Verification items for the finished model (mm, model axes). A direction names the side the tool comes from. Coordinates: 2 decimals unless noted, no trailing zeros. Order: outer loops, then holes, each group sorted by start corner. A loop starts at its lowest first (then second) coordinate and runs counter-clockwise, first axis right, second up. Notation, with made-up numbers: (65.25, -30.5) -> (109.25, -30.5) arc R21 cw to (109.25, 6.5) -> close; hole circle Ø5 at (78, 18). An arc over 180 degrees is marked (long way). Write item = value, one per line. Start each with the question number.
1. Thickness scan on line 1 along X through (y, z) = (29.5, 60); line 2 along Y through (x, z) = (66, 35); line 3 along Y through (x, z) = (14.5, 46.5). Record the ranges inside material, lowest first. Write a range as from..to.
2. Cross-section at C-C on y = 9. Record the cut outline in (x, z).
3. Cross-section at D-D on z = 33.5. Record the cut outline in (x, y).
4. Go/stop test with flat-tipped pins: P1, Ø5, axis at y = 49, z = 34.5, coming from the +X side; P2, Ø8.5, axis at x = 60, z = 7.5, coming from the +Y side; P3, Ø2, axis at x = 39.5, z = 43.5, coming from the +Y side; P4, Ø5, axis at x = 5.5, y = 64.5, coming from the +Z side. Record where each tip stops, or that it passes through.
5. Cross-section at B-B on x = 50.5. Record the cut outline in (y, z), plus the area to 3 significant figures.
6. Cross-section at A-A on z = 63. Record the cut outline in (x, y).
7. Release check for a two-part mould opening along X. For faces 1 (the flat face through (38.1, 57, 30)), 2 (the flat face through (35, 19, 38.1)), 3 (the flat face through (21.59, 57, 35)) record: +X half, -X half, draft (parallel to the pull), parting line (faces both ways), or undercut.
8. Set-up check for faces 4 (the flat face through (38.1, 8, 57)), 5 (the flat face through (35, 38.1, 19)), 6 (the flat face through (38.1, 57, 8)): record each of +Z, -Z, +X, -X, +Y, -Y from which the full face is reachable in a straight line by a thin tool's end or side.
Autodesk Inventor part; units mm, degrees
ref_plane "YZ Plane" through (0, 0, 0) normal (1, 0, 0) x (0, 1, 0)
ref_plane "XZ Plane" through (0, 0, 0) normal (0, 1, 0) x (-1, 0, 0)
ref_plane "XY Plane" through (0, 0, 0) normal (0, 0, 1) x (1, 0, 0)
sketch "Sketch1" plane through (0, 0, 0) normal (0, 0, 1) x (1, 0, 0)
  line L0 (0, 0) -> (38.1, 0)
  line L1 (38.1, 0) -> (38.1, 38.1)
  line L2 (38.1, 38.1) -> (0, 38.1)
  line L3 (0, 38.1) -> (0, 0)
  dimension "d0" = 38.1
  dimension "d1" = 38.1
extrude "Extrusion1" add sketch "Sketch1" along normal blind 38.1
sketch "Sketch2" plane through (0, 0, 38.1) normal (0, 0, 1) x (1, 0, 0)
  line L0 (6.35, 6.35) -> (32.004, 6.35)
  line L1 (32.004, 6.35) -> (32.004, 32.004)
  line L2 (32.004, 32.004) -> (6.35, 32.004)
  line L3 (6.35, 32.004) -> (6.35, 6.35)
  line L4 (38.1, 0) -> (38.1, 38.1)
  line L5 (0, 0) -> (38.1, 0)
  line L6 (38.1, 0) -> (38.1, 38.1)
  line L7 (38.1, 38.1) -> (0, 38.1)
  line L8 (0, 38.1) -> (0, 0)
  dimension "d4" = 25.654
  dimension "d5" = 25.654
extrude "Extrusion2" cut sketch "Sketch2" against normal blind 31.75 contours L3 L2 L1 L0
sketch "Sketch5" plane through (0, 0, 38.1) normal (0, 0, 1) x (1, 0, 0)
  line L0 (6.35, 6.35) -> (6.35, 32.004)
  line L1 (6.35, 6.35) -> (32.004, 6.35)
  line L2 (32.004, 6.35) -> (32.004, 32.004)
  line L3 (32.004, 32.004) -> (6.35, 32.004)
  line L4 (6.35, 32.004) -> (6.35, 6.35)
  line L5 (0, 0) -> (38.1, 0)
  line L6 (0, 0) -> (38.1, 0)
  line L7 (38.1, 0) -> (38.1, 38.1)
  line L8 (38.1, 38.1) -> (0, 38.1)
  line L9 (0, 38.1) -> (0, 0)
extrude "Extrusion4" add sketch "Sketch5" along normal blind 38.1
sketch "Sketch7" plane through (38.1, 0, 0) normal (1, 0, 0) x (0, 0, -1)
  line L0 (0, 0) -> (-76.2, 0)
  line L1 (0, 0) -> (-38.1, 0)
  line L2 (-38.1, 0) -> (-38.1, 38.1)
  line L3 (-38.1, 38.1) -> (0, 38.1)
  line L4 (0, 38.1) -> (0, 0)
  line L5 (-76.2, 6.35) -> (-6.35, 6.35)
  line L6 (-6.35, 6.35) -> (-32.004, 6.35)
  line L7 (-32.004, 6.35) -> (-32.004, 32.004)
  line L8 (-32.004, 32.004) -> (-6.35, 32.004)
  line L9 (-6.35, 32.004) -> (-6.35, 6.35)
  dimension "d16" = 38.1
  dimension "d17" = 38.1
  dimension "d20" = 25.654
  dimension "d21" = 25.654
extrude "Extrusion6" add sketch "Sketch7" along normal blind 38.1
sketch "Sketch9" plane through (38.1, 6.35, 6.35) normal (1, 0, 0) x (0, 0, -1)
  line L0 (-25.654, 0) -> (-25.654, 25.654)
  line L1 (0, 0) -> (0, 25.654)
  line L2 (-25.654, 0) -> (0, 0)
  line L3 (0, 0) -> (0, 25.654)
  line L4 (0, 25.654) -> (-25.654, 25.654)
  line L5 (-25.654, 25.654) -> (-25.654, 0)
  point P0 (6.35, -6.35)
extrude "Extrusion7" cut sketch "Sketch9" against normal blind 31.75
sketch "Sketch10" plane through (0, 38.1, 76.2) normal (0, 1, 0) x (1, 0, 0)
  line L0 (76.2, 69.85) -> (6.35, 69.85)
  line L1 (6.35, 69.85) -> (32.004, 69.85)
  line L2 (32.004, 69.85) -> (32.004, 44.196)
  line L3 (32.004, 44.196) -> (6.35, 44.196)
  line L4 (6.35, 44.196) -> (6.35, 69.85)
  line L5 (38.1, 38.1) -> (38.1, 0)
  line L6 (0, 76.2) -> (0, 0)
  line L7 (38.1, 38.1) -> (0, 38.1)
  line L8 (0, 38.1) -> (0, 76.2)
  line L9 (0, 76.2) -> (38.1, 76.2)
  line L10 (38.1, 76.2) -> (38.1, 38.1)
  point P0 (0, 38.1)
  dimension "d26" = 25.654
  dimension "d27" = 25.654
extrude "Extrusion8" add sketch "Sketch10" along normal blind 38.1
sketch "Sketch11" plane through (6.35, 38.1, 6.35) normal (0, 1, 0) x (1, 0, 0)
  line L0 (0, -25.654) -> (25.654, -25.654)
  line L1 (25.654, -25.654) -> (0, -25.654)
  line L2 (0, -25.654) -> (0, 0)
  line L3 (0, 0) -> (25.654, 0)
  line L4 (25.654, 0) -> (25.654, -25.654)
  point P0 (-6.35, 6.35)
extrude "Extrusion9" cut sketch "Sketch11" against normal blind 6.35
sketch "Sketch12" plane through (0, 76.2, 76.2) normal (0, 1, 0) x (1, 0, 0)
  line L0 (38.1, 55.88) -> (32.004, 55.88)
  line L1 (32.004, 55.88) -> (32.004, 58.42)
  line L2 (32.004, 58.42) -> (38.1, 58.42)
  line L3 (38.1, 58.42) -> (38.1, 55.88)
  point P0 (0, 76.2)
  dimension "d32" = 6.096
  dimension "d33" = 2.54
extrude "Extrusion10" cut sketch "Sketch12" against normal blind 38.1
sketch "Sketch13" plane through (76.2, 38.1, 38.1) normal (0, 1, 0) x (1, 0, 0)
  line L0 (0, 31.75) -> (0, 6.096)
  line L1 (-44.196, 17.78) -> (0, 17.78)
  line L2 (0, 17.78) -> (0, 20.32)
  line L3 (0, 20.32) -> (-44.196, 20.32)
  line L4 (-44.196, 20.32) -> (-44.196, 17.78)
  point P0 (-76.2, 38.1)
  dimension "d36" = 2.54
extrude "Extrusion11" cut sketch "Sketch13" against normal blind 6.35
sketch "Sketch15" plane through (0, 76.2, 76.2) normal (0, 1, 0) x (1, 0, 0)
  line L0 (17.78, 38.1) -> (20.32, 38.1)
  line L1 (20.32, 38.1) -> (20.32, 44.196)
  line L2 (20.32, 44.196) -> (17.78, 44.196)
  line L3 (17.78, 44.196) -> (17.78, 38.1)
  point P0 (0, 76.2)
  dimension "d39" = 2.54
  dimension "d40" = 6.096
extrude "Extrusion12" cut sketch "Sketch15" against normal blind 38.1
sketch "Sketch16" plane through (0, 38.1, 76.2) normal (0, 1, 0) x (1, 0, 0)
  line L0 (20.32, 44.196) -> (20.32, 38.1)
  line L1 (0, 0) -> (38.1, 0)
  line L2 (20.32, 44.196) -> (17.78, 44.196)
  line L3 (17.78, 44.196) -> (17.78, 0)
  line L4 (17.78, 0) -> (20.32, 0)
  line L5 (20.32, 0) -> (20.32, 44.196)
  point P0 (0, 76.2)
  dimension "d43" = 2.54
extrude "Extrusion13" cut sketch "Sketch16" against normal blind 6.35
sketch "Sketch17" plane through (38.1, 0, 76.2) normal (1, 0, 0) x (0, 0, -1)
  line L0 (38.1, 0) -> (38.1, 38.1)
  line L1 (0, 17.78) -> (38.1, 17.78)
  line L2 (38.1, 17.78) -> (38.1, 20.32)
  line L3 (38.1, 20.32) -> (0, 20.32)
  line L4 (0, 20.32) -> (0, 17.78)
  point P0 (76.2, 0)
  dimension "d46" = 2.54
extrude "Extrusion14" cut sketch "Sketch17" against normal blind 6.35
sketch "Sketch18" plane through (38.1, 0, 38.1) normal (0, 0, 1) x (1, 0, 0)
  line L0 (0, 17.78) -> (38.1, 17.78)
  line L1 (38.1, 17.78) -> (38.1, 20.32)
  line L2 (38.1, 20.32) -> (0, 20.32)
  line L3 (0, 20.32) -> (0, 17.78)
  point P0 (-38.1, 0)
  dimension "d49" = 38.1
  dimension "d50" = 2.54
extrude "Extrusion15" cut sketch "Sketch18" against normal blind 6.35
sketch "Sketch20" plane through (38.1, 38.1, 38.1) normal (0, 0, 1) x (1, 0, 0)
  line L0 (-17.78, -6.096) -> (-17.78, 38.1)
  line L1 (0, 0) -> (-17.78, 0)
  line L2 (-17.78, 38.1) -> (-16.51, 38.1)
  line L3 (-16.51, 38.1) -> (-16.51, 0)
  line L4 (-16.51, 0) -> (-17.78, 0)
  line L5 (-17.78, 0) -> (-17.78, 38.1)
  point P0 (-38.1, -38.1)
  dimension "d53" = 1.27
extrude "Extrusion16" cut sketch "Sketch20" against normal blind 6.35
sketch "Sketch21" plane through (38.1, 38.1, 76.2) normal (0, 1, 0) x (1, 0, 0)
  line L0 (-17.78, 0) -> (-17.78, 44.196)
  line L1 (0, 0) -> (-17.78, 0)
  line L2 (-17.78, 44.196) -> (-16.51, 44.196)
  line L3 (-16.51, 44.196) -> (-16.51, 0)
  line L4 (-16.51, 0) -> (-17.78, 0)
  line L5 (-17.78, 0) -> (-17.78, 44.196)
  point P0 (-38.1, 76.2)
  dimension "d56" = 1.27
extrude "Extrusion17" cut sketch "Sketch21" against normal blind 6.35
sketch "Sketch23" plane through (0, 38.1, 38.1) normal (0, 0, 1) x (1, 0, 0)
  line L0 (17.78, 0) -> (17.78, 38.1)
  line L1 (17.78, 0) -> (0, 0)
  line L2 (17.78, 38.1) -> (16.51, 38.1)
  line L3 (16.51, 38.1) -> (16.51, 0)
  line L4 (16.51, 0) -> (17.78, 0)
  line L5 (17.78, 0) -> (17.78, 38.1)
  point P0 (0, -38.1)
  dimension "d59" = 1.27
extrude "Extrusion18" cut sketch "Sketch23" against normal blind 6.35
sketch "Sketch24" plane through (0, 38.1, 76.2) normal (0, 1, 0) x (1, 0, 0)
  line L0 (17.78, 44.196) -> (17.78, 0)
  line L1 (17.78, 0) -> (0, 0)
  line L2 (17.78, 44.196) -> (16.51, 44.196)
  line L3 (16.51, 44.196) -> (16.51, 0)
  line L4 (16.51, 0) -> (17.78, 0)
  line L5 (17.78, 0) -> (17.78, 44.196)
  point P0 (0, 76.2)
  dimension "d62" = 1.27
extrude "Extrusion19" cut sketch "Sketch24" against normal blind 6.35
sketch "Sketch25" plane through (38.1, 0, 76.2) normal (1, 0, 0) x (0, 0, -1)
  line L0 (38.1, 0) -> (38.1, 17.78)
  line L1 (38.1, 17.78) -> (0, 17.78)
  line L2 (0, 17.78) -> (0, 16.51)
  line L3 (0, 16.51) -> (38.1, 16.51)
  line L4 (38.1, 16.51) -> (38.1, 17.78)
  point P0 (76.2, 0)
  dimension "d65" = 38.1
  dimension "d66" = 1.27
extrude "Extrusion20" cut sketch "Sketch25" against normal blind 6.35
sketch "Sketch26" plane through (38.1, 38.1, 76.2) normal (1, 0, 0) x (0, 0, -1)
  line L0 (0, -17.78) -> (38.1, -17.78)
  line L1 (38.1, -17.78) -> (0, -17.78)
  line L2 (0, -17.78) -> (0, -16.51)
  line L3 (0, -16.51) -> (38.1, -16.51)
  line L4 (38.1, -16.51) -> (38.1, -17.78)
  point P0 (76.2, -38.1)
  dimension "d69" = 38.1
  dimension "d70" = 1.27
extrude "Extrusion21" cut sketch "Sketch26" against normal blind 6.35
sketch "Sketch27" plane through (38.1, 0, 38.1) normal (0, 0, 1) x (1, 0, 0)
  line L0 (0, 21.59) -> (0, 38.1)
  line L1 (0, 20.32) -> (38.1, 20.32)
  line L2 (0, 21.59) -> (38.1, 21.59)
  line L3 (38.1, 21.59) -> (38.1, 20.32)
  line L4 (38.1, 20.32) -> (0, 20.32)
  line L5 (0, 20.32) -> (0, 21.59)
  line L6 (38.1, 17.78) -> (0, 17.78)
  line L7 (0, 17.78) -> (38.1, 17.78)
  line L8 (38.1, 17.78) -> (38.1, 16.51)
  line L9 (38.1, 16.51) -> (0, 16.51)
  line L10 (0, 16.51) -> (0, 17.78)
  point P0 (-38.1, 0)
  dimension "d73" = 38.1
  dimension "d74" = 1.27
extrude "Extrusion22" cut sketch "Sketch27" against normal blind 6.35
sketch "Sketch28" plane through (38.1, 38.1, 38.1) normal (0, 1, 0) x (1, 0, 0)
  line L0 (0, 20.32) -> (38.1, 20.32)
  line L1 (0, 20.32) -> (38.1, 20.32)
  line L2 (38.1, 20.32) -> (38.1, 21.59)
  line L3 (38.1, 21.59) -> (0, 21.59)
  line L4 (0, 21.59) -> (0, 20.32)
  line L5 (-6.096, 17.78) -> (38.1, 17.78)
  line L6 (38.1, 17.78) -> (0, 17.78)
  line L7 (0, 17.78) -> (0, 16.51)
  line L8 (0, 16.51) -> (38.1, 16.51)
  line L9 (38.1, 16.51) -> (38.1, 17.78)
  point P0 (-38.1, 38.1)
  point P1 (0, 17.78)
  dimension "d77" = 38.1
  dimension "d78" = 1.27
  dimension "d79" = 38.1
  dimension "d80" = 1.27
extrude "Extrusion23" cut sketch "Sketch28" against normal blind 6.35
sketch "Sketch29" plane through (38.1, 38.1, 0) normal (1, 0, 0) x (0, 0, -1)
  line L0 (-17.78, -6.096) -> (-6.35, -6.096)
  line L1 (-6.35, 38.1) -> (-17.78, 38.1)
  line L2 (-17.78, -6.096) -> (-16.51, -6.096)
  line L3 (-16.51, -6.096) -> (-16.51, 38.1)
  line L4 (-16.51, 38.1) -> (-17.78, 38.1)
  line L5 (-17.78, 38.1) -> (-17.78, -6.096)
  line L6 (-21.59, 0) -> (-21.59, -6.096)
  line L7 (-20.32, 38.1) -> (-20.32, -6.096)
  line L8 (-21.59, -6.096) -> (-20.32, -6.096)
  line L9 (-20.32, -6.096) -> (-20.32, 38.1)
  line L10 (-20.32, 38.1) -> (-21.59, 38.1)
  line L11 (-21.59, 38.1) -> (-21.59, -6.096)
  point P0 (0, -38.1)
  point P1 (-20.32, -6.096)
  dimension "d83" = 1.27
extrude "Extrusion24" cut sketch "Sketch29" against normal blind 6.35
sketch "Sketch30" plane through (76.2, 38.1, 21.59) normal (0, 0, -1) x (-1, 0, 0)
  line L0 (0, 0) -> (38.1, 0)
  line L1 (44.196, 38.1) -> (44.196, -6.096)
  line L2 (38.1, 0) -> (44.196, 0)
  line L3 (44.196, 0) -> (44.196, -6.096)
  line L4 (44.196, -6.096) -> (38.1, -6.096)
  line L5 (38.1, -6.096) -> (38.1, 0)
  point P0 (76.2, -38.1)
  point P1 (44.196, 0)
extrude "Extrusion25" add sketch "Sketch30" along normal blind 5.08
sketch "Sketch31" plane through (21.59, 38.1, 38.1) normal (-1, 0, 0) x (0, 0, 1)
  line L0 (38.1, -6.096) -> (-6.096, -6.096)
  line L1 (0, 0) -> (-6.096, 0)
  line L2 (-6.096, 0) -> (-6.096, -6.096)
  line L3 (-6.096, -6.096) -> (0, -6.096)
  line L4 (0, -6.096) -> (0, 0)
  point P0 (-38.1, -38.1)
extrude "Extrusion26" add sketch "Sketch31" along normal blind 5.08
sketch "Sketch32" plane through (0, 0, 76.2) normal (-1, 0, 0) x (0, 0, 1)
  line L0 (0, 38.1) -> (0, 0)
  line L1 (0, 19.05) -> (-76.2, 19.05)
  line L2 (-76.2, 19.05) -> (-76.2, 0)
  line L3 (-76.2, 0) -> (0, 0)
  line L4 (0, 0) -> (0, 19.05)
  line L5 (-76.2, 0) -> (-56.896, 0)
  line L6 (-56.896, 0) -> (-56.896, 76.2)
  line L7 (-56.896, 76.2) -> (-76.2, 76.2)
  line L8 (-76.2, 76.2) -> (-76.2, 0)
  point P0 (0, 0)
  point P1 (-56.896, 19.05)
  dimension "d90" = 19.304
  dimension "d91" = 76.2
extrude "Extrusion27" add sketch "Sketch32" along normal blind 12.7
sketch "Sketch33" plane through (-12.7, 0, 76.2) normal (-1, 0, 0) x (0, 0, 1)
  line L0 (-56.896, 19.05) -> (0, 19.05)
  line L1 (-56.896, 19.05) -> (0, 19.05)
  line L2 (0, 19.05) -> (0, 76.2)
  line L3 (0, 76.2) -> (-56.896, 76.2)
  line L4 (-56.896, 76.2) -> (-56.896, 19.05)
  line L5 (-38.1, 38.1) -> (-38.1, 76.2)
  line L6 (0, 76.2) -> (-38.1, 76.2)
  line L7 (-38.1, 76.2) -> (-38.1, 38.1)
  line L8 (-38.1, 38.1) -> (0, 38.1)
  line L9 (0, 38.1) -> (0, 76.2)
  point P0 (-76.2, 0)
  dimension "d94" = 56.896
  dimension "d95" = 57.15
extrude "Extrusion28" add sketch "Sketch33" against normal blind 6.35 contours L4 L3 L5 L8 L2 L0
properties part number "corner connector w rail (back)"
Worked out:
q1.line_1 = -12.7..-6.35, 0..6.35, 32..38.1
q1.line_2 = 0..16.51, 21.59..38.1
q1.line_3 = 0..6.35, 32..38.1
q2.outline = (-12.7, 0) -> (76.2, 0) -> (76.2, 6.35) -> (6.35, 6.35) -> (6.35, 76.2) -> (-12.7, 76.2) -> close; (32, 32) -> (76.2, 32) -> (76.2, 38.1) -> (38.1, 38.1) -> (38.1, 76.2) -> (32, 76.2) -> close
q3.outline = (-12.7, 0) -> (76.2, 0) -> (76.2, 16.51) -> (38.1, 16.51) -> (38.1, 21.59) -> (76.2, 21.59) -> (76.2, 38.1) -> (38.1, 38.1) -> (38.1, 76.2) -> (21.59, 76.2) -> (21.59, 38.1) -> (16.51, 38.1) -> (16.51, 76.2) -> (0, 76.2) -> (0, 19.05) -> (-6.35, 19.05) -> (-6.35, 76.2) -> (-12.7, 76.2) -> close; hole (6.35, 6.35) -> (32, 6.35) -> (32, 32) -> (6.35, 32) -> close
q4.P1 = 38.1
q4.P2 = 38.1
q4.P3 = through
q4.P4 = 38.1
q5.outline = (0, 0) -> (38.1, 0) -> (38.1, 16.51) -> (32, 16.51) -> (32, 6.35) -> (6.35, 6.35) -> (6.35, 32) -> (16.51, 32) -> (16.51, 38.1) -> (0, 38.1) -> close; (21.59, 32) -> (32, 32) -> (32, 21.59) -> (38.1, 21.59) -> (38.1, 38.1) -> (21.59, 38.1) -> close
q5.area = 732 mm²
q6.outline = (-12.7, 0) -> (38.1, 0) -> (38.1, 16.51) -> (32, 16.51) -> (32, 6.35) -> (6.35, 6.35) -> (6.35, 32) -> (16.51, 32) -> (16.51, 38.1) -> (0, 38.1) -> (0, 19.05) -> (-6.35, 19.05) -> (-6.35, 38.1) -> (-12.7, 38.1) -> close; (21.59, 32) -> (32, 32) -> (32, 21.59) -> (38.1, 21.59) -> (38.1, 38.1) -> (21.59, 38.1) -> close
q7.face_1 = +X half
q7.face_2 = draft
q7.face_3 = undercut
q8.face_4 = +Z, +X, +Y, -Y
q8.face_5 = +X, +Y
q8.face_6 = +Z, -Z, +X, +Y
